```python
from build123d import *

# Parameters (mm, degrees)
SKETCH044_R        = 1.6
POCKET029_DEPTH    = 14.001
POCKET030_DEPTH    = 1
CHAMFER026025_SIZE = 0.99


with BuildPart() as part:
    # Sketch043 → Revolution001 (revolve)
    with BuildSketch(Plane.YZ):
        Polygon((-6.05, 0), (-6.05, 10.5), (0, 10.5), (0, 14), (-25, 14), (-25, 7), (-22, 7), (-21, 8), (-15, 8), (-14, 7), (-9.05, 7), (-7.05, 0), align=None)
    revolve(axis=Axis((0, 0, 0), (0, 0, 1)))

    # Sketch044 (on Face3 of Revolution001) → Pocket029 (cut, through all)
    with BuildSketch(Plane(origin=(0, 0, 14), x_dir=(0, -1, 0), z_dir=(0, 0, 1))):
        with Locations((-3, 0)):
            Circle(SKETCH044_R)
        with Locations((3, 0)):
            Circle(SKETCH044_R)
    extrude(amount=-POCKET029_DEPTH, mode=Mode.SUBTRACT)

    # Sketch045 (on Face8 of Pocket029) → Pocket030 (cut)
    with BuildSketch(Plane(origin=(0, 0, 14), x_dir=(0, -1, 0), z_dir=(0, 0, 1))):
        with BuildLine():
            ThreePointArc((-3, 3.2), (-6.2, 0), (-3, -3.2))
            Line((-3, -3.2), (3, -3.2))
            ThreePointArc((3, -3.2), (6.2, 0), (3, 3.2))
            Line((-3, 3.2), (3, 3.2))
        make_face()
    extrude(amount=-POCKET030_DEPTH, mode=Mode.SUBTRACT)

    # Chamfer026025
    chamfer026025_edges = [part.edges().sort_by_distance(p)[0] for p in [
        (0, -6.2, 14),
        (-3.2, 0, 14),
        (0, 6.2, 14),
        (3.2, 0, 14),
    ]]
    chamfer(chamfer026025_edges, length=CHAMFER026025_SIZE)


with BuildPart() as part_1:
    # Body001001001002003010002 placement: moved
    add(part.part.moved(Location((0, 0, 45))))


solid = part_1.part
```
The listing builds one solid part. Answer for the finished solid, in the listing's coordinates (mm). A direction names the side the tool comes from. Coordinates: 2 decimals unless noted, no trailing zeros. Write each loop counter-clockwise with the first axis right and the second up, starting at its lowest first coordinate (ties: lowest second). Pieces come first, ordered by that corner, then holes.
Q1. Given P1, Ø7.5, axis at x = 0, y = 0, coming from the -Z side; P2, Ø5, axis at y = -9, z = 52, coming from the -X side; P3, Ø2, axis at x = -0.5, z = 55.5, coming from the +Y side; P4, Ø5, axis at x = -5, z = 57, coming from the -Y side, each flat-ended and moving along its own axis, determine where each tip first touches the part or whether it passes through.
Returned:
P1: stops at z = 55.5
P2: stops at x = -24.14
P3: stops at y = 25
P4: stops at y = -24.87
Q2. Section C-C, the plane z = 56.25 is taken. Write down the section's boundary in (x, y), then the cut area to 3 significant figures.
Returned:
outline: circle Ø50 at (0, 0); hole circle Ø3.2 at (0, -3); hole circle Ø3.2 at (0, 3)
area: 1,950 mm2
Q3. Section A-A, the plane x = 0 is taken. Give the number of separate pieces and of enclosed holes in the cut face, then the cut area to 3 significant figures.
Returned:
separate pieces: 3
enclosed holes: 0
area: 292 mm2
Q4. Find the intervals of material crossed by line 1 along X through (y, z) = (0, 53.75); line 2 along Z through (x, y) = (10.5, 18); line 3 along X through (y, z) = (0, 49.5), in increasing order.
Returned:
line 1: x = -25 to -6.05, 6.05 to 25
line 2: z = 53 to 59
line 3: x = -8.34 to -6.05, 6.05 to 8.34
Q5. Which of the six approach directions +Z, -Z, +X, -X, +Y, -Y give full straight-line access (tool end or side, diameter ignored) to faces 1 (the cylindrical face through (0.07, -1.4, 56.77)), 2 (the flat face through (0, 0, 58)), 3 (the cylindrical face through (-2.317, -5.589, 50.324))?
Returned:
face 1: +Z, -Z
face 2: +Z
face 3: -Z
Q6. The mould has two halves that part along Y. Classify faces 4 (the flat face through (-14, -9, 53)), 5 (the conical face through (7.307, 0.959, 46.118)), 6 (the flat face through (-5, 0, 59)): released by +Y, released by -Y, zero draft, split by the parting line, or undercut.
Returned:
face 4: undercut
face 5: split by the parting line
face 6: zero draft
Q7. Section D-D, the plane z = 50.5 is taken. Write down the section's boundary in (x, y).
Returned:
outline: circle Ø17.24 at (0, 0); hole circle Ø12.1 at (0, 0)
